Autodesk Inventor part; units mm, degrees
ref_plane "YZ Plane" through (0, 0, 0) normal (1, 0, 0) x (0, 1, 0)
ref_plane "XZ Plane" through (0, 0, 0) normal (0, 1, 0) x (-1, 0, 0)
ref_plane "XY Plane" through (0, 0, 0) normal (0, 0, 1) x (1, 0, 0)
sketch "Sketch1" plane through (0, 0, 0) normal (0, 0, 1) x (1, 0, 0)
  circle A0 centre (0, 0) radius 6
  dimension "d0" = 12
extrude "Extrusion1" add sketch "Sketch1" along normal blind 19
sketch "Sketch2" plane through (0, 0, 19) normal (0, 0, 1) x (1, 0, 0)
  circle A0 centre (0, 0) radius 6
  circle A1 centre (0, 0) radius 3.1
  dimension "d3" = 6.2
extrude "Extrusion2" cut sketch "Sketch2" against normal blind 19 contours A1
chamfer "Chamfer1" distance 0.5 angle 45 4 edges at (-6, 0, 19) (-3.1, 0, 19) (-3.1, 0, 0) (-6, 0, 0)
properties part number "6mmLinearBearing"
Geometry check sheet. Reference: the model listing, model coordinates, mm. Coordinates: 2 decimals unless noted, no trailing zeros. Order: outer loops, then holes, each group sorted by start corner. A loop starts at its lowest first (then second) coordinate and runs counter-clockwise, first axis right, second up. Notation, with made-up numbers: M 13.5,89 L 49.5,89 A23 ccw 49.5,113 Z; hole C 29,39 d11. An arc over 180 degrees is marked long. Use CSV: the item, a comma, the result in double quotes.
Item 1: Mould release check, pull along Y, two halves, no side actions. Record for faces 1 (the flat face through (4, -1, 0)), 2 (the cylindrical face through (-6, 0, 9)), 3 (the cylindrical face through (1.43, -2.75, 9.63)): pulls with the +Y half, pulls with the -Y half, needs draft (parallel to the pull), parting line crosses it, or undercut.
Returned:
face 1,"needs draft"
face 2,"parting line crosses it"
face 3,"undercut"
Item 2: Cross-section at A-A on y = 0. Record the cut outline in (x, z), then the cut area to 3 significant figures.
Returned:
outline,"M -6,0.5 L -5.5,0 L -3.6,0 L -3.1,0.5 L -3.1,18.5 L -3.6,19 L -5.5,19 L -6,18.5 Z; M 3.1,0.5 L 3.6,0 L 5.5,0 L 6,0.5 L 6,18.5 L 5.5,19 L 3.6,19 L 3.1,18.5 Z"
area,"109 mm2"
Item 3: Cross-section at C-C on z = 3.5. Record the cut outline in (x, y).
Returned:
outline,"C 0,0 d12; hole C 0,0 d6.2"
Item 4: Thickness scan on line 1 along Y through (x, z) = (0, 12.25); line 2 along X through (y, z) = (-1.5, 6); line 3 along Y through (x, z) = (-0.75, 18). Record the ranges inside material, lowest first.
Returned:
line 1,"y = -6 to -3.1, 3.1 to 6"
line 2,"x = -5.81 to -2.71, 2.71 to 5.81"
line 3,"y = -5.95 to -3.01, 3.01 to 5.95"
Item 5: Gauge pin test, flat ends, axial feed: pin 1 Ø6 at (x, z) = (-4.5, 11) entering from -Y; pin 2 Ø1.5 at (x, y) = (0, 2.5) entering from -Z; pin 3 Ø5 at (x, y) = (0, 0) entering from +Z; pin 4 Ø4 at (x, z) = (-4, 15) entering from +Y. Record the tip position at first contact, or that the pin passes through.
Returned:
pin 1,"stops at y = -5.81"
pin 2,"stops at z = 0.35"
pin 3,"passes through"
pin 4,"stops at y = 5.66"
